For this review, take the finished solid that the model builds, in its own axes (mm). Face numbers are marked on the shaded views. A direction names the side the tool comes from. Round coordinates to 2 decimals unless told otherwise and drop trailing zeros. Order: outer loops, then holes, each group sorted by start corner. A loop starts at its lowest first (then second) coordinate and runs counter-clockwise, first axis right, second up. Notation, with made-up numbers: (-36, -37) -> (3, -37) arc R29 cw to (3, -12) -> close; hole circle Ø11 at (-3, 24). An arc over 180 degrees is marked (long way). Use a Markdown table: item, result. Add a question column.
1) Machinability: for the marked faces 4, 5, 6 and 7, which of the approach directions +Z, -Z, +X, -X, +Y, -Y give a long, thin tool a straight path to every point of the face, cutting with its end or side? Answer none if there is none.
2) Wall thickness on line 1 along X through (y, z) = (2.5, 0); line 2 along Y through (x, z) = (-8.85, 15); line 3 along Y through (x, z) = (-8.5, -2.5): over which ranges is each line inside the solid? List them lowest first. Write a range as [from, to].
3) Consider section C-C (x = 16). State the section outline as (y, z) points, plus the area to 3 significant figures.
4) Draft analysis for pull direction X (two halves, no side actions). For the marked faces 1, 2 and 3, state which applies: pulls with the +X half, pulls with the -X half, needs draft (parallel to the pull), parting line crosses it, or undercut.
5) Consider section B-B (z = 0). State the section outline as (x, y) points.
6) Clearance check with flat-ended pins moving along their axes: P1, Ø2.5, axis at x = -8, z = 8, coming from the +Y side; P2, Ø2, axis at y = 0, z = 10.5, coming from the +X side; P3, Ø6, axis at y = -15, z = 17.5, coming from the -X side. State where each tip first meets the part, or that it passes through.
7) Consider section A-A (y = -10). State the section outline as (x, z) points.
8) Consider section D-D (y = -3.5). State the section outline as (x, z) points, plus the area to 3 significant figures.
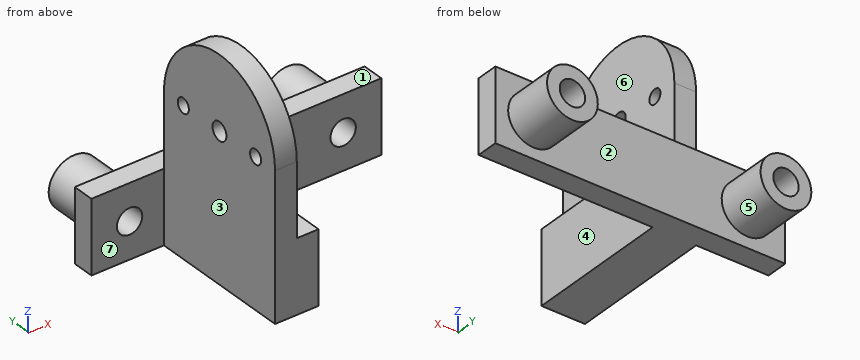
```python
from build123d import *

# Parameters (mm, degrees)
SKETCH_1_W      = 40
SKETCH_1_H      = 10
SKETCH_1_R      = 1.75
EXTRUDE_1_DEPTH = 3
EXTRUDE_START   = -10
SKETCH_2_R      = 1
SKETCH_2_R_2    = 1.25
EXTRUDE_2_DEPTH = 3
SKETCH_3_W      = 3
SKETCH_3_H      = 10
EXTRUDE_3_DEPTH = 20
SKETCH_4_R      = 3.5
SKETCH_4_R_2    = 1.75
EXTRUDE_4_DEPTH = 7


with BuildPart() as part:
    # 草图1 → 凸台-拉伸1 (new body)
    with BuildSketch(Plane(origin=(0, 0, 0), x_dir=(1, 0, 0), z_dir=(0, 1, 0))):
        Rectangle(SKETCH_1_W, SKETCH_1_H)
        with Locations(Location((-14.732, 0, 0), (0, 0, 270))):
            Circle(SKETCH_1_R, mode=Mode.SUBTRACT)
        with Locations(Location((14.732, 0, 0), (0, 0, 270))):
            Circle(SKETCH_1_R, mode=Mode.SUBTRACT)
    extrude(amount=EXTRUDE_1_DEPTH)

    # 草图2 → 凸台-拉伸2 (add)
    with BuildSketch(Plane(origin=(0, 0, 0), x_dir=(0, 0, -1), z_dir=(1, 0, 0)).offset(EXTRUDE_START)):
        with BuildLine():
            Line((5, 0), (-15, 0))
            ThreePointArc((-15, 0), (-25, -10), (-15, -20))
            Line((-15, -20), (5, -20))
            Line((5, -20), (5, 0))
        make_face()
        with Locations((-15, -3.5)):
            Circle(SKETCH_2_R, mode=Mode.SUBTRACT)
        with Locations((-15, -16.5)):
            Circle(SKETCH_2_R, mode=Mode.SUBTRACT)
        with Locations((-15, -10)):
            Circle(SKETCH_2_R_2, mode=Mode.SUBTRACT)
    extrude(amount=EXTRUDE_2_DEPTH)

    # 草图3 → 凸台-拉伸3 (add)
    with BuildSketch(Plane.XZ):
        with Locations((-5.5, 0)):
            Rectangle(SKETCH_3_W, SKETCH_3_H)
    extrude(amount=EXTRUDE_3_DEPTH)

    # 草图4 → 凸台-拉伸4 (add)
    # profile 1 of 2: a face of its own
    with BuildSketch(Plane(origin=(0, 3, 0), x_dir=(1, 0, 0), z_dir=(0, 1, 0))):
        with Locations(Location((-14.732, 0, 0), (0, 0, 270))):
            Circle(SKETCH_4_R)
        with Locations(Location((-14.732, 0, 0), (0, 0, 270))):
            Circle(SKETCH_4_R_2, mode=Mode.SUBTRACT)
    # profile 2 of 2: a face of its own
    with BuildSketch(Plane(origin=(0, 3, 0), x_dir=(1, 0, 0), z_dir=(0, 1, 0))):
        with Locations(Location((14.732, 0, 0), (0, 0, 90))):
            Circle(SKETCH_4_R)
        with Locations(Location((14.732, 0, 0), (0, 0, 270))):
            Circle(SKETCH_4_R_2, mode=Mode.SUBTRACT)
    extrude(amount=EXTRUDE_4_DEPTH)


solid = part.part
```
Results list:
| question | item | result |
|---|---|---|
| 1 | face 4 | +Z, -Z, +X, -Y |
| 1 | face 5 | +Y |
| 1 | face 6 | +Z, +X, +Y, -Y |
| 1 | face 7 | +Z, -Z, -X, -Y |
| 2 | line 1 | [-20, -16.48], [-12.98, 12.98], [16.48, 20] |
| 2 | line 2 | [-20, -17.5], [-15.5, -11.25], [-8.75, -4.5], [-2.5, 0] |
| 2 | line 3 | [-20, 3] |
| 3 | outline | (0, -5) -> (3, -5) -> (3, -3.26) -> (10, -3.26) -> (10, -1.21) -> (0, -1.21) -> close; (0, 1.21) -> (10, 1.21) -> (10, 3.26) -> (3, 3.26) -> (3, 5) -> (0, 5) -> close |
| 3 | area | 51.5 mm2 |
| 4 | face 1 | needs draft |
| 4 | face 2 | undercut |
| 4 | face 3 | pulls with the -X half |
| 5 | outline | (-20, 0) -> (-16.48, 0) -> (-16.48, 10) -> (-18.23, 10) -> (-18.23, 3) -> (-20, 3) -> close; (-12.98, 0) -> (-10, 0) -> (-10, -20) -> (-4, -20) -> (-4, 0) -> (12.98, 0) -> (12.98, 10) -> (11.23, 10) -> (11.23, 3) -> (-11.23, 3) -> (-11.23, 10) -> (-12.98, 10) -> close; (16.48, 0) -> (20, 0) -> (20, 3) -> (18.23, 3) -> (18.23, 10) -> (16.48, 10) -> close |
| 6 | P1 | y = 0 |
| 6 | P2 | x = -7 |
| 6 | P3 | x = -10 |
| 7 | outline | (-10, -5) -> (-4, -5) -> (-4, 5) -> (-7, 5) -> (-7, 13.75) -> (-10, 13.75) -> close; (-10, 16.25) -> (-7, 16.25) -> (-7, 25) -> (-10, 25) -> close |
| 8 | outline | (-10, -5) -> (-4, -5) -> (-4, 5) -> (-7, 5) -> (-7, 14) -> (-10, 14) -> close; (-10, 16) -> (-7, 16) -> (-7, 22.6) -> (-10, 22.6) -> close |
| 8 | area | 107 mm2 |
